Source: CAD feature listing. Evaluate the final solid. Frame: model axes, mm. Round coordinates to 2 decimals unless told otherwise and drop trailing zeros. Write each loop counter-clockwise with the first axis right and the second up, starting at its lowest first coordinate (ties: lowest second). Pieces come first, ordered by that corner, then holes. Notation, with made-up numbers: M 34,-30 L 73,-30 A18 ccw 73,-13 Z; hole C 32,40 d8. An arc over 180 degrees is marked long. Answer in a Markdown table with one row per item.
Autodesk Inventor part; units mm, degrees
ref_plane "YZ Plane" through (0, 0, 0) normal (1, 0, 0) x (0, 1, 0)
ref_plane "XZ Plane" through (0, 0, 0) normal (0, 1, 0) x (-1, 0, 0)
ref_plane "XY Plane" through (0, 0, 0) normal (0, 0, 1) x (1, 0, 0)
sketch "Sketch1" plane through (0, 0, 0) normal (0, 0, 1) x (1, 0, 0)
  line L0 (0, 0) -> (20, 0)
  line L1 (20, 0) -> (20, 17.5)
  line L2 (20, 17.5) -> (0, 17.5)
  line L3 (0, 17.5) -> (0, 0)
  dimension "d0" = 20
  dimension "d1" = 17.5
extrude "Extrusion1" add sketch "Sketch1" along normal blind 250
sketch "Sketch2" plane through (0, 17.5, 0) normal (0, 1, 0) x (1, 0, 0)
  circle A0 centre (10, -20) radius 3
  line L0 (20, 0) -> (0, 0)
  point P0 (10, 0)
  dimension "d4" = 6
  dimension "d5" = 20
extrude "Extrusion2" cut sketch "Sketch2" against normal up to surface (17.5 mm away)
sketch "Sketch3" plane through (0, 17.5, 0) normal (0, 1, 0) x (1, 0, 0)
  circle A0 centre (10, -20) radius 4.75
  circle A1 centre (10, -20) radius 3 construction
  point P0 (0, 0)
  dimension "d8" = 9.5
extrude "Extrusion3" cut sketch "Sketch3" against normal blind 8.5
pattern_linear "Rectangular Pattern1" count 18 spacing 60 along (0, 0, 1) of "Extrusion2", "Extrusion3"
properties part number "HGW20CC_Rack"
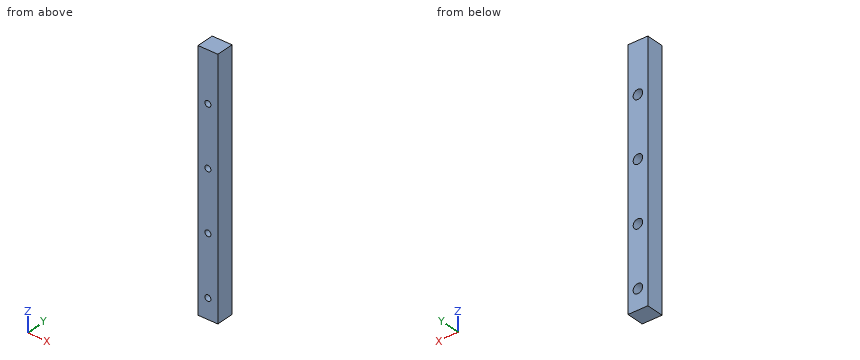
Q1. Material intervals for probe 1 along Z at (x, y) = (10, 14.25); probe 2 along Z at (x, y) = (10, 6.5); probe 3 along X at (y, z) = (11.25, 140), sorted ascending.
Solutions:
| item | result |
|---|---|
| probe 1 | z = 0 to 15.25, 24.75 to 75.25, 84.75 to 135.25, 144.75 to 195.25, 204.75 to 250 |
| probe 2 | z = 0 to 17, 23 to 77, 83 to 137, 143 to 197, 203 to 250 |
| probe 3 | x = 0 to 5.25, 14.75 to 20 |
Q2. Section A-A (y = 11.5). Return loops of the section in (x, z).
Solutions:
| item | result |
|---|---|
| outline | M 0,0 L 20,0 L 20,250 L 0,250 Z; hole C 10,20 d9.5; hole C 10,80 d9.5; hole C 10,140 d9.5; hole C 10,200 d9.5 |
Q3. Section C-C (x = 10). State how many separate pieces and enclosed holes the cut face has, and give its area (3 significant figures).
Solutions:
| item | result |
|---|---|
| separate pieces | 5 |
| enclosed holes | 0 |
| area | 3,840 mm2 |
Q4. Contact query for a flat-ended pin moving along its axis: pin 1 Ø5 at (x, z) = (10.5, 19.5) entering from +Y. Output: stop coordinate, or through.
Solutions:
| item | result |
|---|---|
| pin 1 | stops at y = 9 |
Q5. Section D-D (y = 2.25). Return loops of the section in (x, z).
Solutions:
| item | result |
|---|---|
| outline | M 0,0 L 20,0 L 20,250 L 0,250 Z; hole C 10,20 d6; hole C 10,80 d6; hole C 10,140 d6; hole C 10,200 d6 |
Q6. Section B-B (z = 20). Return loops of the section in (x, y), and give its area (3 significant figures).
Solutions:
| item | result |
|---|---|
| outline | M 0,0 L 7,0 L 7,9 L 5.25,9 L 5.25,17.5 L 0,17.5 Z; M 13,0 L 20,0 L 20,17.5 L 14.75,17.5 L 14.75,9 L 13,9 Z |
| area | 215 mm2 |
